Here's the drawing with two shaded views (mm, measured from the low corner). I have some questions. A direction names the side the tool comes from. Give positions to 0.01 mm unless a question says otherwise; leave off trailing zeros. Order: outer loops, then holes, each group sorted by start corner. A loop starts at its lowest first (then second) coordinate and runs counter-clockwise, first axis right, second up. Notation, with made-up numbers: (68, 84.25) - (107, 84.25) arc R28 ccw to (107, 118.25) - close; hole circle Ø11 at (24, 40.25). An arc over 180 degrees is marked (long way). Use one line per item in the form item = value. Start each with the question number.
1) Suppose I cut it at A-A, the plane x = 8.5. Write out the boundary of the cut face in (y, z), and give its area (3 significant figures).
2) Which directions (+Z, -Z, +X, -X, +Y, -Y) give clear straight access to the entire face, cutting with the end or side of a thin tool? Please do the marked faces 1, 2 and 3.
3) Please list where these lines run through material, in increasing order: probe 1 along Y at (x, z) = (8.5, 8.3); probe 2 along Y at (x, z) = (8.25, 14); probe 3 along X at (y, z) = (21, 2.5).
4) Suppose I cut it at C-C, the plane y = 2. Write out the boundary of the cut face in (x, z), and give its area (3 significant figures).
5) Suppose I cut it at D-D, the plane y = 48. Write out the boundary of the cut face in (x, z).
6) For pin 1 (5 mm diameter, centred on x = 8.5, z = 4.5, fed in from -Y); pin 2 (1.2 mm diameter, centred on x = 8, y = 6, fed in from +Z); pin 3 (4 mm diameter, centred on x = 8, y = 20, fed in from -Z), each with a flat end and sliding along its axis, tell me the tip position at first contact or that it passes through.
7) Suppose I cut it at B-B, the plane z = 8.5. Write out the boundary of the cut face in (x, y), and give its area (3 significant figures).
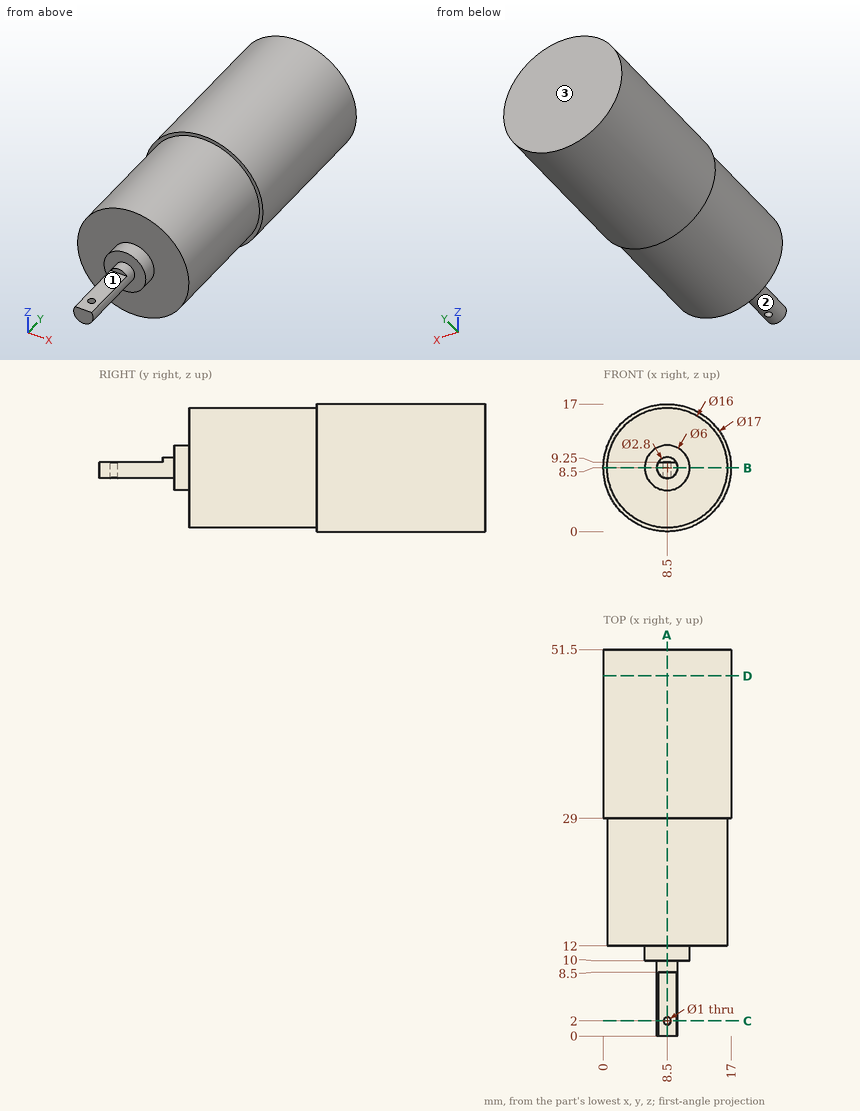
Result sheet:
q1.outline = (0, 7.1) - (1.5, 7.1) - (1.5, 9.25) - (0, 9.25) - close; (2.5, 7.1) - (10, 7.1) - (10, 5.5) - (12, 5.5) - (12, 0.5) - (29, 0.5) - (29, 0) - (51.5, 0) - (51.5, 17) - (29, 17) - (29, 16.5) - (12, 16.5) - (12, 11.5) - (10, 11.5) - (10, 9.9) - (8.5, 9.9) - (8.5, 9.25) - (2.5, 9.25) - close
q1.area = 687 mm²
q2.face_1 = +Z, +X, -X, -Y
q2.face_2 = -Y
q2.face_3 = +Z, -Z, +X, -X, +Y
q3.probe_1 = 0 to 1.5, 2.5 to 51.5
q3.probe_2 = 12 to 51.5
q3.probe_3 = 3.21 to 13.79
q4.outline = (7.32, 9.25) arc R1.4 ccw to (8, 7.19) - (8, 9.25) - close; (9, 7.19) arc R1.4 ccw to (9.68, 9.25) - (9, 9.25) - close
q4.area = 2.95 mm²
q5.outline = circle Ø17 at (8.5, 8.5)
q6.pin_1 = 10
q6.pin_2 = 9.25
q6.pin_3 = 0.5
q7.outline = (0, 29) - (0.5, 29) - (0.5, 12) - (5.5, 12) - (5.5, 10) - (7.1, 10) - (7.1, 0) - (9.9, 0) - (9.9, 10) - (11.5, 10) - (11.5, 12) - (16.5, 12) - (16.5, 29) - (17, 29) - (17, 51.5) - (0, 51.5) - close; hole circle Ø1 at (8.5, 2)
q7.area = 694 mm²
